Read the model definition and answer for the solid it produces. Units are mm, in the model's axes. Coordinates: 2 decimals unless noted, no trailing zeros. Order: outer loops, then holes, each group sorted by start corner. A loop starts at its lowest first (then second) coordinate and runs counter-clockwise, first axis right, second up. Notation, with made-up numbers: (76, -23) -> (132, -23) arc R22 cw to (132, -6) -> close; hole circle Ø5 at (-8, -9). An arc over 180 degrees is marked (long way). Answer in a Markdown table with one row per item.
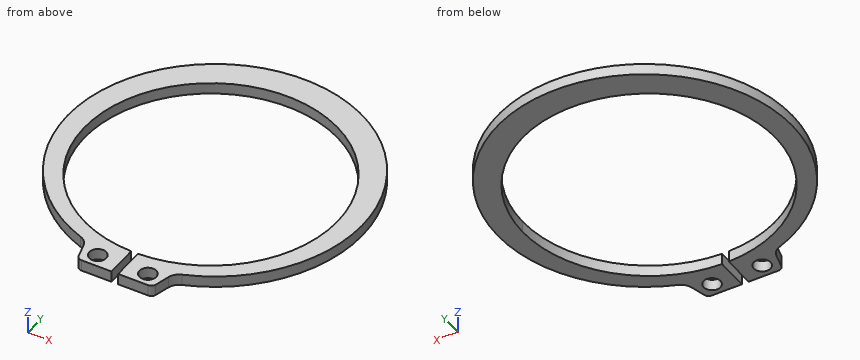
from build123d import *

# Parameters (mm, degrees)
BASE_SKETCH_R    = 11.9888
BASE_SKETCH_R_2  = 0.8001
BASE_DEPTH       = 1.0668
CUT_SKETCH_W     = 0.635
CUT_SKETCH_H     = 7.458306792
BOTTOM_CUT_DEPTH = 22.059418629


with BuildPart() as part:
    # Base Sketch → Base (new body)
    with BuildSketch(Plane.XY):
        with BuildLine():
            Line((-3.16619789, -15.7226), (3.16619789, -15.7226))
            ThreePointArc((3.16619789, -15.7226), (3.475448696, -15.617623497), (3.65688821, -15.346080075))
            Line((3.65688821, -15.346080075), (4.023345402, -13.978443217))
            ThreePointArc((4.023345402, -13.978443217), (4.312600377, -13.450377126), (4.812565268, -13.114881454))
            ThreePointArc((4.812565268, -13.114881454), (0, 13.97), (-4.812565268, -13.114881454))
            ThreePointArc((-4.812565268, -13.114881454), (-4.312600377, -13.450377126), (-4.023345402, -13.978443217))
            Line((-4.023345402, -13.978443217), (-3.65688821, -15.346080075))
            ThreePointArc((-3.65688821, -15.346080075), (-3.475448696, -15.617623497), (-3.16619789, -15.7226))
        make_face()
        with Locations((0, -0.635)):
            Circle(BASE_SKETCH_R, mode=Mode.SUBTRACT)
        with Locations((2.3749, -14.4526)):
            Circle(BASE_SKETCH_R_2, mode=Mode.SUBTRACT)
        with Locations((-2.3749, -14.4526)):
            Circle(BASE_SKETCH_R_2, mode=Mode.SUBTRACT)
    extrude(amount=BASE_DEPTH)

    # Cut Sketch → Bottom Cut (cut, through all)
    with BuildSketch(Plane.XY.offset(1.0668)):
        with Locations((0, -12.6238)):
            Rectangle(CUT_SKETCH_W, CUT_SKETCH_H)
    extrude(amount=-BOTTOM_CUT_DEPTH, mode=Mode.SUBTRACT)


solid = part.part
Q1. Consider line 1 (X direction, y = -14, z = 1); line 2 (X direction, y = 6.5, z = 0.6); line 3 (Y direction, x = 4.25, z = 0.65). Determine where each line is inside the solid, lowest interval first.
Outcome:
| item | result |
|---|---|
| line 1 | -4.02 to -3.03, -1.72 to -0.32, 0.32 to 1.72, 3.03 to 4.02 |
| line 2 | -12.37 to -9.63, 9.63 to 12.37 |
| line 3 | -13.52 to -11.85, 10.58 to 13.31 |
Q2. The part is cut by section B-B (x = 7.5). Write down the section's boundary in (y, z), then the cut area to 3 significant figures.
Outcome:
| item | result |
|---|---|
| outline | (-11.79, 0) -> (-9.99, 0) -> (-9.99, 1.07) -> (-11.79, 1.07) -> close; (8.72, 0) -> (11.79, 0) -> (11.79, 1.07) -> (8.72, 1.07) -> close |
| area | 5.19 mm² |
Q3. The part is cut by section C-C (z = 0.7). Write down the section's boundary in (x, y) (1 decimal).
Outcome:
| item | result |
|---|---|
| outline | (-4.8, -13.1) arc R1.3 cw to (-4, -14) -> (-3.7, -15.3) arc R0.5 ccw to (-3.2, -15.7) -> (-0.3, -15.7) -> (-0.3, -12.6) arc R12 cw (long way) to (0.3, -12.6) -> (0.3, -15.7) -> (3.2, -15.7) arc R0.5 ccw to (3.7, -15.3) -> (4, -14) arc R1.3 cw to (4.8, -13.1) arc R14 ccw (long way) to start; hole circle Ø1.6 at (-2.4, -14.5); hole circle Ø1.6 at (2.4, -14.5) |
Q4. The part is cut by section A-A (y = 10.5). Write down the section's boundary in (x, z), then the cut area to 3 significant figures.
Outcome:
| item | result |
|---|---|
| outline | (-9.21, 0) -> (-4.44, 0) -> (-4.44, 1.07) -> (-9.21, 1.07) -> close; (4.44, 0) -> (9.21, 0) -> (9.21, 1.07) -> (4.44, 1.07) -> close |
| area | 10.2 mm² |
